```python
from build123d import *

# Parameters (mm, degrees)
ESQUISSE1_W        = 250
ESQUISSE1_H        = 50
BOSS_EXTRU_1_DEPTH = 2
BOSS_EXTRU_2_DEPTH = 250


with BuildPart() as part:
    # Esquisse1 → Boss.-Extru.1 (new body)
    with BuildSketch(Plane.XY):
        with Locations((-125, 25)):
            Rectangle(ESQUISSE1_W, ESQUISSE1_H)
    extrude(amount=BOSS_EXTRU_1_DEPTH)

    # Esquisse2 → Boss.-Extru.2 (add)
    with BuildSketch(Plane(origin=(0, 0, 0), x_dir=(0, 0, -1), z_dir=(1, 0, 0))):
        Polygon((-2, 0), (-17, 0), (-7, 2.5), (-2, 2.5), align=None)
    extrude(amount=-BOSS_EXTRU_2_DEPTH)


solid = part.part
```
The model under review builds one solid part; all positions refer to its coordinate system, in mm. A direction names the side the tool comes from. Give positions to 0.01 mm unless a question says otherwise; leave off trailing zeros. Write each loop counter-clockwise with the first axis right and the second up, starting at its lowest first coordinate (ties: lowest second). Pieces come first, ordered by that corner, then holes. Notation, with made-up numbers: (80.25, -1.5) -> (136.25, -1.5) arc R17 ccw to (136.25, 29.5) -> close; hole circle Ø8 at (-15, 73.5). An arc over 180 degrees is marked (long way). Answer in a Markdown table with one row per item.
1) For L1, parallel to Z at x = -44, y = 34; L2, parallel to Y at x = -104.5, z = 3.5; L3, parallel to Y at x = -98, z = 10.75, list the stretches that pass through material, from the lowest coordinate up. Write a range as [from, to].
Worked answers:
| item | result |
|---|---|
| L1 | [0, 2] |
| L2 | [0, 2.5] |
| L3 | [0, 1.56] |
2) Add section A-A on x = -162. State the section outline as (y, z) points.
Worked answers:
| item | result |
|---|---|
| outline | (0, 0) -> (50, 0) -> (50, 2) -> (2.5, 2) -> (2.5, 7) -> (0, 17) -> close |
3) Add section C-C on z = 9.5. State the section outline as (x, y) points (3 decimals), plus the area to 3 significant figures.
Worked answers:
| item | result |
|---|---|
| outline | (-250, 0) -> (0, 0) -> (0, 1.875) -> (-250, 1.875) -> close |
| area | 469 mm² |
4) Clearance check with flat-ended pins moving along their axes: P1, Ø1.5, axis at y = 21, z = 3, coming from the -X side; P2, Ø14, axis at x = -179.5, y = 15.5, coming from the +Z side; P3, Ø1.5, axis at x = -170, z = 5, coming from the +Y side. State where each tip first meets the part, or that it passes through.
Worked answers:
| item | result |
|---|---|
| P1 | through |
| P2 | z = 2 |
| P3 | y = 2.5 |
5) Tool access review of faces 1 (the flat face through (-123, 2.5, 5)), 2 (the flat face through (-123, 0, 8)): name each direction out of +Z, -Z, +X, -X, +Y, -Y from which nothing blocks a thin tool from reaching the whole face with its end or side.
Worked answers:
| item | result |
|---|---|
| face 1 | +Z, +X, -X, +Y |
| face 2 | +Z, -Z, +X, -X, -Y |
6) Add section B-B on y = 31.5. State the section outline as (x, z) points.
Worked answers:
| item | result |
|---|---|
| outline | (-250, 0) -> (0, 0) -> (0, 2) -> (-250, 2) -> close |
